CAD build for the part. Positions are in the model's coordinates, mm. Round coordinates to 2 decimals unless told otherwise and drop trailing zeros. Order: outer loops, then holes, each group sorted by start corner. A loop starts at its lowest first (then second) coordinate and runs counter-clockwise, first axis right, second up. Notation, with made-up numbers: M -36.75,-27.75 L -26.75,-27.75 A20 ccw -26.75,-0.75 Z; hole C 28.25,29 d10. An arc over 180 degrees is marked long. Answer as a JSON object with one key per item and string values.
Autodesk Inventor part; units mm, degrees
ref_plane "YZ Plane" through (0, 0, 0) normal (1, 0, 0) x (0, 1, 0)
ref_plane "XZ Plane" through (0, 0, 0) normal (0, 1, 0) x (-1, 0, 0)
ref_plane "XY Plane" through (0, 0, 0) normal (0, 0, 1) x (1, 0, 0)
sketch "Sketch1" plane through (0, 0, 0) normal (0, 0, 1) x (1, 0, 0)
  line L0 (0, 0) -> (0, 50)
  line L1 (0, 50) -> (20, 50)
  line L2 (20, 50) -> (20, 90)
  line L3 (20, 90) -> (420, 90)
  line L4 (420, 90) -> (420, 50)
  line L5 (420, 50) -> (440, 50)
  line L6 (440, 50) -> (440, 0)
  line L7 (440, 0) -> (0, 0)
  circle A0 centre (220, 60) radius 10
  circle A1 centre (80, 35) radius 6
  circle A2 centre (360, 35) radius 6
  circle A3 centre (80, 35) radius 50
  circle A4 centre (130, 35) radius 6
  circle A5 centre (310, 35) radius 6
  dimension "d1" = 50
  dimension "d2" = 20
  dimension "d3" = 40
  dimension "d4" = 400
  dimension "d5" = 40
  dimension "d6" = 20
  dimension "d7" = 20
  dimension "d8" = 12
  dimension "d9" = 12
  dimension "d10" = 80
  dimension "d11" = 80
  dimension "d12" = 35
  dimension "d13" = 35
  dimension "d14" = 30
  dimension "d17" = 100
  dimension "d18" = 12
  dimension "d19" = 12
  dimension "d20" = 130
  dimension "d21" = 130
  dimension "d22" = 35
  dimension "d23" = 35
extrude "Extrusion1" add sketch "Sketch1" along normal blind 5 contours L0 L1 L2 L3 L4 L5 L6 L7 A3 A4 | A3 A4 L7 | A4 A3 | A3 A4 | A5
properties part number "sUPORTE1"
Item 1: Saw through at A-A on x = 220. List the corners of the cut face in (y, z), and give its area (3 significant figures).
Worked answers:
{"outline": "M 0,0 L 50,0 L 50,5 L 0,5 Z; M 70,0 L 90,0 L 90,5 L 70,5 Z", "area": "350 mm2"}
Item 2: Saw through at D-D on y = 60. List the corners of the cut face in (x, z), and give its area (3 significant figures).
Worked answers:
{"outline": "M 20,0 L 210,0 L 210,5 L 20,5 Z; M 230,0 L 420,0 L 420,5 L 230,5 Z", "area": "1,900 mm2"}
Item 3: Two-plate mould, pull along Y, no slides. Class faces 1 (the cylindrical face through (229.237, 63.83, 2.465)), 2 (the flat face through (217, 46, 0)): released by +Y, released by -Y, zero draft, split by the parting line, or undercut.
Worked answers:
{"face 1": "undercut", "face 2": "zero draft"}
Item 4: Saw through at C-C on z = 1.8. List the corners of the cut face in (x, y), and give its area (3 significant figures).
Worked answers:
{"outline": "M 0,0 L 440,0 L 440,50 L 420,50 L 420,90 L 20,90 L 20,50 L 0,50 Z; hole C 80,35 d12; hole C 220,60 d20; hole C 360,35 d12", "area": "37,500 mm2"}
Item 5: Wall check: line 1 along X through (y, z) = (35.5, 3.15); line 2 along Y through (x, z) = (220, 3); line 3 along X through (y, z) = (29.5, 4.6). Give the ranges that are in metal, low to high. Write a range as [from, to].
Worked answers:
{"line 1": "x = [0, 74.02], [85.98, 354.02], [365.98, 440]", "line 2": "y = [0, 50], [70, 90]", "line 3": "x = [0, 77.6], [82.4, 357.6], [362.4, 440]"}
Item 6: Saw through at B-B on y = 35. List the corners of the cut face in (x, z), and give its area (3 significant figures).
Worked answers:
{"outline": "M 0,0 L 74,0 L 74,5 L 0,5 Z; M 86,0 L 354,0 L 354,5 L 86,5 Z; M 366,0 L 440,0 L 440,5 L 366,5 Z", "area": "2,080 mm2"}
Item 7: Drop flat-ended pins along their axis: pin 1 Ø1.5 at (y, z) = (71.5, 2) entering from -X; pin 2 Ø3 at (x, z) = (368, 1.5) entering from -Y; pin 3 Ø2.5 at (x, z) = (431, 3.5) entering from +Y. Give the stop position or say it passes through.
Worked answers:
{"pin 1": "stops at x = 20", "pin 2": "stops at y = 0", "pin 3": "stops at y = 50"}
